The listing builds one solid part. Answer for the finished solid, in the listing's coordinates (mm). Round coordinates to 2 decimals unless told otherwise and drop trailing zeros. Write each loop counter-clockwise with the first axis right and the second up, starting at its lowest first coordinate (ties: lowest second). Pieces come first, ordered by that corner, then holes. Notation, with made-up numbers: (-7.75, 62.5) - (20.25, 62.5) arc R20 ccw to (20.25, 68.5) - close; hole circle Ø11 at (28.5, -13.5). An arc over 180 degrees is marked (long way). Use a Markdown table: item, result. Add a question column.
1) A cutting plane is placed at A-A (x = -2). Give the vertices of the cut face in (y, z), then the cut area to 3 significant figures.
2) A cutting plane is placed at B-B (y = 0.8). Give the vertices of the cut face in (x, z), then the cut area to 3 significant figures.
3) A cutting plane is placed at C-C (x = 18). Give the vertices of the cut face in (y, z).
4) A cutting plane is placed at D-D (z = 7). Give the vertices of the cut face in (x, y).
5) Each of these flat-tipped pins is pushed along its axis until it touches: P1, Ø0.6, axis at y = 1, z = -9.5, coming from the +X side; P2, Ø8, axis at x = -10, z = -13, coming from the -Y side. Where does it stop, or does it pass through?
6) Find the intervals of material crossed by probe 1 along Z at (x, y) = (-10.5, 1.8); probe 2 along X at (y, z) = (1.1, 5.5); probe 3 along X at (y, z) = (0.9, -9.5), in increasing order. Write a range as from..to.
```python
from build123d import *

# Parameters (mm, degrees)
BOSS_EXTRUDE1_DEPTH = 2


with BuildPart() as part:
    # Sketch2 → Boss-Extrude1 (new body)
    with BuildSketch(Plane(origin=(0, 0, 0), x_dir=(1, 0, 0), z_dir=(0, 1, 0))):
        with BuildLine():
            Line((20, 20), (20, 16))
            Line((20, 16), (-16, 16))
            Line((-16, 16), (-16, 2))
            Line((-16, 2), (16, 2))
            ThreePointArc((16, 2), (18.828427125, 0.828427125), (20, -2))
            Line((20, -2), (20, -16))
            ThreePointArc((20, -16), (18.828427125, -18.828427125), (16, -20))
            Line((16, -20), (-20, -20))
            Line((-20, -20), (-20, -16))
            Line((-20, -16), (16, -16))
            Line((16, -16), (16, -2))
            Line((16, -2), (-16, -2))
            ThreePointArc((-16, -2), (-18.828427125, -0.828427125), (-20, 2))
            Line((-20, 2), (-20, 16))
            ThreePointArc((-20, 16), (-18.828427125, 18.828427125), (-16, 20))
            Line((-16, 20), (20, 20))
        make_face()
    extrude(amount=BOSS_EXTRUDE1_DEPTH)


solid = part.part
```
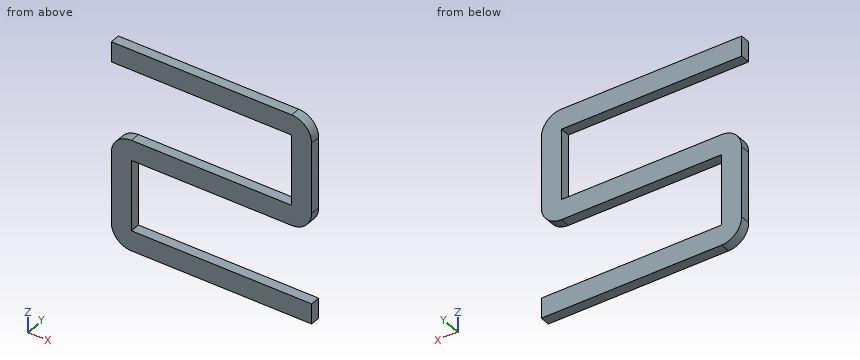
Entries:
| question | item | result |
|---|---|---|
| 1 | outline | (0, -20) - (2, -20) - (2, -16) - (0, -16) - close; (0, -2) - (2, -2) - (2, 2) - (0, 2) - close; (0, 16) - (2, 16) - (2, 20) - (0, 20) - close |
| 1 | area | 24.0 mm² |
| 2 | outline | (-20, -16) arc R4 ccw to (-16, -20) - (20, -20) - (20, -16) - (-16, -16) - (-16, -2) - (16, -2) arc R4 ccw to (20, 2) - (20, 16) arc R4 ccw to (16, 20) - (-20, 20) - (-20, 16) - (16, 16) - (16, 2) - (-16, 2) arc R4 ccw to (-20, -2) - close |
| 2 | area | 578 mm² |
| 3 | outline | (0, -20) - (2, -20) - (2, -16) - (0, -16) - close; (0, -1.46) - (2, -1.46) - (2, 19.46) - (0, 19.46) - close |
| 4 | outline | (16, 0) - (20, 0) - (20, 2) - (16, 2) - close |
| 5 | P1 | stops at x = -16 |
| 5 | P2 | stops at y = 0 |
| 6 | probe 1 | z = -20..-16, -2..2, 16..20 |
| 6 | probe 2 | x = 16..20 |
| 6 | probe 3 | x = -20..-16 |
